For this review, take the finished solid that the model builds, in its own axes (mm). Give positions to 0.01 mm unless a question says otherwise; leave off trailing zeros. Write each loop counter-clockwise with the first axis right and the second up, starting at its lowest first coordinate (ties: lowest second). Pieces come first, ordered by that corner, then holes. Notation, with made-up numbers: (0.25, -3) -> (15.25, -3) arc R28 cw to (15.25, 18) -> close; hole circle Ø6 at (-6.5, -16). An arc over 180 degrees is marked (long way). Return JSON: item names as keys, results as strings.
from build123d import *

# Parameters (mm, degrees)
F0_W      = 800
F0_H      = 150
F1_DEPTH  = 12.5
F2_W      = 10
F2_H      = 10
F3_DEPTH  = 15
F4_R      = 2.5
F5_DEPTH  = 10
F6_SIZE   = 1
F7_R      = 2.5
F8_DEPTH  = 10
F9_R      = 2.5
F10_DEPTH = 10
F11_R     = 2.5
F12_DEPTH = 10
F13_R     = 2.5
F14_DEPTH = 10
F15_SIZE  = 1


with BuildPart() as f1:
    # F0 (on Top) → F1 (new body)
    with BuildSketch(Plane.XY):
        Rectangle(F0_W, F0_H)
    extrude(amount=F1_DEPTH)

    # F2 (on face) → F3 (join)
    with BuildSketch(Plane.XY.offset(12.5)):
        with Locations((-302, -40)):
            Rectangle(F2_W, F2_H)
        with Locations((-163, -40)):
            Rectangle(F2_W, F2_H)
        with Locations((-87.5, -40)):
            Rectangle(F2_W, F2_H)
        with Locations((90.5, -40)):
            Rectangle(F2_W, F2_H)
        with Locations((256.5, -40)):
            Rectangle(F2_W, F2_H)
    extrude(amount=F3_DEPTH)

    # F4 (on face) → F5 (join)
    with BuildSketch(Plane.XY.offset(27.5)):
        with Locations((-302, -40)):
            Circle(F4_R)
    extrude(amount=F5_DEPTH)

    # F6
    f6_edges = [f1.edges().sort_by_distance(p)[0] for p in [
        (-304.5, -40, 37.5),
    ]]
    chamfer(f6_edges, length=F6_SIZE)

    # F7 (on face) → F8 (join)
    with BuildSketch(Plane.XY.offset(27.5)):
        with Locations((-163, -40)):
            Circle(F7_R)
    extrude(amount=F8_DEPTH)

    # F9 (on face) → F10 (join)
    with BuildSketch(Plane.XY.offset(27.5)):
        with Locations((-87.5, -40)):
            Circle(F9_R)
    extrude(amount=F10_DEPTH)

    # F11 (on face) → F12 (join)
    with BuildSketch(Plane.XY.offset(27.5)):
        with Locations((90.5, -40)):
            Circle(F11_R)
    extrude(amount=F12_DEPTH)

    # F13 (on face) → F14 (join)
    with BuildSketch(Plane.XY.offset(27.5)):
        with Locations((256.5, -40)):
            Circle(F13_R)
    extrude(amount=F14_DEPTH)

    # F15
    f15_edges = [f1.edges().sort_by_distance(p)[0] for p in [
        (254, -40, 37.5),
        (88, -40, 37.5),
        (-90, -40, 37.5),
        (-165.5, -40, 37.5),
    ]]
    chamfer(f15_edges, length=F15_SIZE)


solid = f1.part
1. To check wall thickness, follow probe 1 along X at (y, z) = (-40, 15); probe 2 along Z at (x, y) = (-331.5, 16.5); probe 3 along Y at (x, z) = (-87, 27). State the ranges of each line that lie inside material, in increasing order.
Results found:
{"probe 1": "x = -307 to -297, -168 to -158, -92.5 to -82.5, 85.5 to 95.5, 251.5 to 261.5", "probe 2": "z = 0 to 12.5", "probe 3": "y = -45 to -35"}
2. For pin 1 (5 mm diameter, centred on x = 90.5, z = 23.5, fed in from +Y); pin 2 (8 mm diameter, centred on y = -37.5, z = 17.5, fed in from +X); pin 3 (11 mm diameter, centred on x = -87, z = 19.5, fed in from -Y), all flat-tipped, find the tip position at first contact; note any pin that passes through.
Results found:
{"pin 1": "stops at y = -35", "pin 2": "stops at x = 261.5", "pin 3": "stops at y = -45"}
3. Add section A-A, the plane y = 5.5. State the section outline as (x, z) points, plus the area to 3 significant figures.
Results found:
{"outline": "(-400, 0) -> (400, 0) -> (400, 12.5) -> (-400, 12.5) -> close", "area": "10,000 mm²"}
4. Add section B-B, the plane x = 37. State the section outline as (y, z) points, plus the area to 4 significant figures.
Results found:
{"outline": "(-75, 0) -> (75, 0) -> (75, 12.5) -> (-75, 12.5) -> close", "area": "1,875 mm²"}
